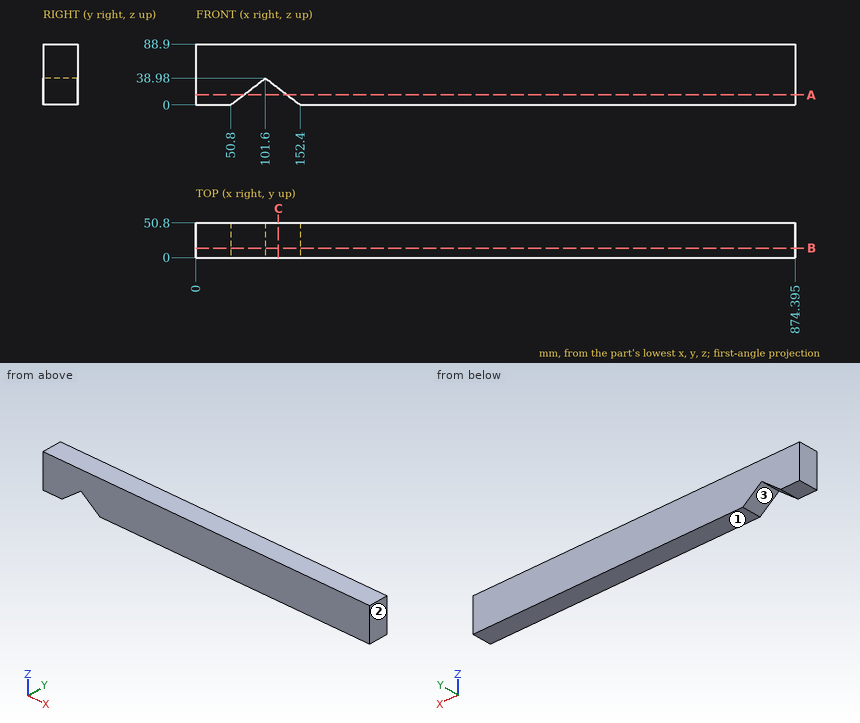
Could you check a few things on this drawing? It's one solid part, dimensions in mm from its lowest x, y, z. Round coordinates to 2 decimals unless told otherwise and drop trailing zeros. Write each loop counter-clockwise with the first axis right and the second up, starting at its lowest first coordinate (ties: lowest second). Pieces come first, ordered by that corner, then holes. Notation, with made-up numbers: (44.5, 10) -> (89.5, 10) arc R29 cw to (89.5, 49) -> close; hole circle Ø1 at (14.25, -1). An arc over 180 degrees is marked (long way). One line per item, written item: value.
1) Suppose I cut it at C-C on x = 120.5. List the corners of the cut face in (y, z) for me.
Filled sheet:
outline: (0, 24.48) -> (50.8, 24.48) -> (50.8, 88.9) -> (0, 88.9) -> close
2) Suppose I cut it at B-B on y = 14. List the corners of the cut face in (x, z) for me (1 decimal), plus the area to 3 significant figures.
Filled sheet:
outline: (0, 0) -> (50.8, 0) -> (101.6, 39) -> (152.4, 0) -> (874.4, 0) -> (874.4, 88.9) -> (0, 88.9) -> close
area: 75,800 mm2
3) I'm going to push a flat-ended pin straight in: pin 1 Ø5 at (x, y) = (92.5, 39) entering from -Z. Where does the tip first touch, or does it pass through?
Filled sheet:
pin 1: stops at z = 30.08
4) If I drill on line 1 (X direction, y = 27.5, z = 14.5) (1 decimal); line 2 (X direction, y = 29, z = 5.5) (1 decimal); line 3 (Z direction, x = 94.5, y = 6), over which ranges is the centre line in solid material (lowest first)? Write a range as [from, to].
Filled sheet:
line 1: x = [0, 69.7], [133.5, 874.4]
line 2: x = [0, 58], [145.2, 874.4]
line 3: z = [33.53, 88.9]
5) Suppose I cut it at A-A on z = 14.5. List the corners of the cut face in (x, y) for me (1 decimal), plus the area to 3 significant figures.
Filled sheet:
outline: (0, 0) -> (69.7, 0) -> (69.7, 50.8) -> (0, 50.8) -> close; (133.5, 0) -> (874.4, 0) -> (874.4, 50.8) -> (133.5, 50.8) -> close
area: 41,200 mm2
6) We'd pull the mould along X, two halves only. Please class the marked faces 1, 2 and 3: released by +X, released by -X, zero draft, split by the parting line, or undercut.
Filled sheet:
face 1: zero draft
face 2: released by +X
face 3: undercut
